Work out the finished part from the listing and answer in its coordinate system (mm). A direction names the side the tool comes from. Coordinates: 2 decimals unless noted, no trailing zeros. Write each loop counter-clockwise with the first axis right and the second up, starting at its lowest first coordinate (ties: lowest second). Pieces come first, ordered by that corner, then holes. Notation, with made-up numbers: (63, 41) - (100, 41) arc R33 cw to (100, 70) - close; hole circle Ø7 at (-33.5, 59.25). An arc over 180 degrees is marked (long way). Answer as a JSON object with one key per item and string values. Group by question number.
from build123d import *

# Parameters (mm, degrees)
SKETCH1_W           = 2.5
SKETCH1_H           = 36.73
SKETCH1_W_2         = 16
SKETCH1_H_2         = 3.175
BOSS_EXTRUDE1_DEPTH = 3.175


with BuildPart() as part:
    # Sketch1 → Boss-Extrude1 (new body)
    with BuildSketch(Plane(origin=(0, 0, 0), x_dir=(1, 0, 0), z_dir=(0, 1, 0))):
        with Locations((-9.25, 0)):
            Rectangle(SKETCH1_W, SKETCH1_H)
        Rectangle(SKETCH1_W_2, SKETCH1_H)
        with Locations((9.25, 0)):
            Rectangle(SKETCH1_W, SKETCH1_H)
        with Locations((0, -19.9525)):
            Rectangle(SKETCH1_W_2, SKETCH1_H_2)
        with Locations((0, 19.9525)):
            Rectangle(SKETCH1_W_2, SKETCH1_H_2)
    extrude(amount=BOSS_EXTRUDE1_DEPTH)


solid = part.part
Q1. A tool of negligible diameter and unlimited length cuts with its end or side. For faces 4 (the face through (-8, 2, 20)), 5 (the face through (9, 2, -18.365)), 6 (the face through (9, 2, 18.365)), 7 (the face through (-9, 2, -18.365)), from which of +Z, -Z, +X, -X, +Y, -Y can it reach the whole face along a straight path? Write none if from no direction.
Q2. Consider L1, parallel to Z at x = 9.25, y = 1.65 (3 decimals); L2, parallel to X at y = 1.7, z = 19.5. Determine where each line is inside the solid, lowest interval first. Write a range as from..to.
Q3. Flat-ended cylindrical pins translate along their axes: pin 1 Ø1 at (y, z) = (1.5, -20) entering from +X; pin 2 Ø1.2 at (x, y) = (-9, 1.5) entering from -Z (3 decimals). Find the tip coordinate at first contact, or state that the pin passes through.
Q4. For a pull along Y with two mould halves and no side action, classify faces 1 (the face through (10.5, 2, 0)), 2 (the face through (0, 0, 0)), 3 (the face through (0, 3.175, 0)) as +Y half, -Y half, draft (parallel to the pull), parting line (faces both ways), or undercut.
Q5. Section A-A on y = 0.7 is taken. Determine the outline of the cut face in (x, z) (3 decimals), plus the area to 3 significant figures.
Numbers:
{
 "1": {"face 4": "+Z, -X, +Y, -Y", "face 5": "-Z, +X, +Y, -Y", "face 6": "+Z, +X, +Y, -Y", "face 7": "-Z, -X, +Y, -Y"},
 "2": {"L1": "z = -18.365..18.365", "L2": "x = -8..8"},
 "3": {"pin 1": "stops at x = 8", "pin 2": "stops at z = -18.365"},
 "4": {"face 1": "draft", "face 2": "-Y half", "face 3": "+Y half"},
 "5": {"outline": "(-10.5, -18.365) - (-8, -18.365) - (-8, -21.54) - (8, -21.54) - (8, -18.365) - (10.5, -18.365) - (10.5, 18.365) - (8, 18.365) - (8, 21.54) - (-8, 21.54) - (-8, 18.365) - (-10.5, 18.365) - close", "area": "873 mm²"}
}
